For this review, take the finished solid that the model builds, in its own axes (mm). A direction names the side the tool comes from. Round coordinates to 2 decimals unless told otherwise and drop trailing zeros. Order: outer loops, then holes, each group sorted by start corner. A loop starts at its lowest first (then second) coordinate and runs counter-clockwise, first axis right, second up. Notation, with made-up numbers: M 57,60 L 79,60 A22 ccw 79,75 Z; hole C 37.5,86 d2. An arc over 180 degrees is marked long. Use a Markdown table: item, result.
from build123d import *

# Parameters (mm, degrees)
SKETCH_1_W               = 205
SKETCH_1_H               = 118
SKETCH_1_R               = 8.5
SKETCH_1_R_2             = 2.5
EXTRUDE_1_DEPTH          = 5
SKETCH_2_W               = 5
SKETCH_2_H               = 20
EXTRUDE_2_DEPTH          = 5
PATTERN_LINEAR_1_COUNT   = 3
PATTERN_LINEAR_1_PITCH   = 40
MIRROR_1_COPY_1_SKETCH_W = 5
MIRROR_1_COPY_1_SKETCH_H = 20
MIRROR_1_COPY_1_DEPTH    = 5
MIRROR_1_COPY_2_SKETCH_W = 5
MIRROR_1_COPY_2_SKETCH_H = 20
MIRROR_1_COPY_2_DEPTH    = 5
SKETCH_3_W               = 20
SKETCH_3_H               = 5
EXTRUDE_3_DEPTH          = 5
PATTERN_LINEAR_2_COUNT   = 3
PATTERN_LINEAR_2_PITCH   = 40
PATTERN_LINEAR_3_COUNT   = 3
PATTERN_LINEAR_3_PITCH   = 40


with BuildPart() as part:
    # 스케치1 → 보스-돌출1 (new body)
    with BuildSketch(Plane.XY):
        Rectangle(SKETCH_1_W, SKETCH_1_H)
        with Locations((48, 4)):
            Circle(SKETCH_1_R, mode=Mode.SUBTRACT)
        with Locations((-48, 4)):
            Circle(SKETCH_1_R, mode=Mode.SUBTRACT)
        with Locations((-74, 4)):
            Circle(SKETCH_1_R_2, mode=Mode.SUBTRACT)
        with Locations(Location((-22, 4, 0), (0, 0, 180))):
            Circle(SKETCH_1_R_2, mode=Mode.SUBTRACT)
        with Locations((22, 4)):
            Circle(SKETCH_1_R_2, mode=Mode.SUBTRACT)
        with Locations(Location((74, 4, 0), (0, 0, 180))):
            Circle(SKETCH_1_R_2, mode=Mode.SUBTRACT)
    extrude(amount=EXTRUDE_1_DEPTH)

    # 스케치2 → 보스-돌출2 (add)
    with BuildSketch(Plane.XY.offset(5)):
        with Locations((-105, -49)):
            Rectangle(SKETCH_2_W, SKETCH_2_H)
    extrude_2 = extrude(amount=-EXTRUDE_2_DEPTH)

    # 선형 패턴1: 보스-돌출2 ×3
    with Locations(*[(0, i * PATTERN_LINEAR_1_PITCH, 0) for i in range(1, PATTERN_LINEAR_1_COUNT)]):
        add(extrude_2)

    # 대칭 복사1: 보스-돌출2 across plane
    add(extrude_2.mirror(Plane(origin=(0, 0, 0), x_dir=(0, 0, 1), z_dir=(1, 0, 0))))

    # 대칭 복사1 copy 1 sketch → 대칭 복사1 copy 1 (add)
    with BuildSketch(Plane(origin=(0, 40, 5), x_dir=(-1, 0, 0), z_dir=(0, 0, 1))):
        with Locations((-105, 49)):
            Rectangle(MIRROR_1_COPY_1_SKETCH_W, MIRROR_1_COPY_1_SKETCH_H)
    extrude(amount=-MIRROR_1_COPY_1_DEPTH)

    # 대칭 복사1 copy 2 sketch → 대칭 복사1 copy 2 (add)
    with BuildSketch(Plane(origin=(0, 80, 5), x_dir=(-1, 0, 0), z_dir=(0, 0, 1))):
        with Locations((-105, 49)):
            Rectangle(MIRROR_1_COPY_2_SKETCH_W, MIRROR_1_COPY_2_SKETCH_H)
    extrude(amount=-MIRROR_1_COPY_2_DEPTH)

    # 스케치3 → 보스-돌출3 (add)
    with BuildSketch(Plane.XY.offset(5)):
        with Locations((0, 61.5)):
            Rectangle(SKETCH_3_W, SKETCH_3_H)
    extrude_3 = extrude(amount=-EXTRUDE_3_DEPTH)

    # 선형 패턴2: 보스-돌출3 ×3
    with Locations(*[(i * PATTERN_LINEAR_2_PITCH, 0, 0) for i in range(1, PATTERN_LINEAR_2_COUNT)]):
        add(extrude_3)

    # 선형 패턴3: 보스-돌출3 ×3
    with Locations(*[(-i * PATTERN_LINEAR_3_PITCH, 0, 0) for i in range(1, PATTERN_LINEAR_3_COUNT)]):
        add(extrude_3)


solid = part.part
Q1. Draft analysis for pull direction Y (two halves, no side actions). For faces 1 (the flat face through (-102.5, 50, 2)), 2 (the flat face through (105, 41, 3)), 3 (the cylindrical face through (76.5, 3.9, 2.5)), state which applies: pulls with the +Y half, pulls with the -Y half, needs draft (parallel to the pull), parting line crosses it, or undercut.
Determined:
| item | result |
|---|---|
| face 1 | needs draft |
| face 2 | pulls with the +Y half |
| face 3 | undercut |
Q2. Add section C-C (x = -22). Write out the cut boundary in (y, z), then the cut area to 3 significant figures.
Determined:
| item | result |
|---|---|
| outline | M -59,0 L 1.5,0 L 1.5,5 L -59,5 Z; M 6.5,0 L 59,0 L 59,5 L 6.5,5 Z |
| area | 565 mm^2 |
Q3. Clearance check with flat-ended pins moving along their axes: pin 1 (2 mm diameter, centred on x = -11.5, z = 1, fed in from +Y); pin 2 (1 mm diameter, centred on y = -22.5, z = 1, fed in from -X); pin 3 (1.5 mm diameter, centred on x = 104, z = 2, fed in from +Y). State where each tip first meets the part, or that it passes through.
Determined:
| item | result |
|---|---|
| pin 1 | stops at y = 59 |
| pin 2 | stops at x = -102.5 |
| pin 3 | stops at y = 41 |
Q4. Add section D-D (y = 51.5). Write out the cut boundary in (x, z).
Determined:
| item | result |
|---|---|
| outline | M -102.5,0 L 102.5,0 L 102.5,5 L -102.5,5 Z |
Q5. Add section B-B (y = 4). Write out the cut boundary in (x, z).
Determined:
| item | result |
|---|---|
| outline | M -102.5,0 L -76.5,0 L -76.5,5 L -102.5,5 Z; M -71.5,0 L -56.5,0 L -56.5,5 L -71.5,5 Z; M -39.5,0 L -24.5,0 L -24.5,5 L -39.5,5 Z; M -19.5,0 L 19.5,0 L 19.5,5 L -19.5,5 Z; M 24.5,0 L 39.5,0 L 39.5,5 L 24.5,5 Z; M 56.5,0 L 71.5,0 L 71.5,5 L 56.5,5 Z; M 76.5,0 L 102.5,0 L 102.5,5 L 76.5,5 Z |
Q6. Machinability: for faces 4 (the flat face through (-30, 61, 3)), 5 (the flat face through (-107.5, 31, 3)), 6 (the flat face through (-105, -19, 3)), 7 (the flat face through (-105, 41, 3)), 8 (the flat face through (102.5, 50, 2)), which of the approach directions +Z, -Z, +X, -X, +Y, -Y give a long, thin tool a straight path to every point of the face, cutting with its end or side? Answer none if there is none.
Determined:
| item | result |
|---|---|
| face 4 | +Z, -Z, +Y |
| face 5 | +Z, -Z, -X, +Y, -Y |
| face 6 | +Z, -Z, -X |
| face 7 | +Z, -Z, -X, +Y |
| face 8 | +Z, -Z, +X, +Y |
Q7. Wall thickness on line 1 along Y through (x, z) = (74, 2.25); line 2 along Y through (x, z) = (-48, 2.5); line 3 along X through (y, z) = (16, 0.9): over which ranges is each line inside the solid? List them lowest first. Write a range as [from, to].
Determined:
| item | result |
|---|---|
| line 1 | y = [-59, 1.5], [6.5, 64] |
| line 2 | y = [-59, -4.5], [12.5, 64] |
| line 3 | x = [-102.5, 102.5] |
Q8. Add section A-A (x = -74). Write out the cut boundary in (y, z).
Determined:
| item | result |
|---|---|
| outline | M -59,0 L 1.5,0 L 1.5,5 L -59,5 Z; M 6.5,0 L 64,0 L 64,5 L 6.5,5 Z |
